from build123d import *

# Parameters (mm, degrees)
SKETCH2_W           = 102
SKETCH2_H           = 96.13
SKETCH2_W_2         = 92
SKETCH2_H_2         = 64.53
BOSS_EXTRUDE1_DEPTH = 85
SKETCH8_R           = 10.25
CUT_EXTRUDE7_DEPTH  = 20
SKETCH9_R           = 12.7
CUT_EXTRUDE8_DEPTH  = 20
SKETCH10_R          = 3.875
CUT_EXTRUDE9_DEPTH  = 142.206388754
SKETCH11_W          = 48.065
SKETCH11_H          = 85
CUT_EXTRUDE10_DEPTH = 142.206388754
SKETCH14_R          = 1.5
BOSS_EXTRUDE2_DEPTH = 10
SKETCH15_R          = 15.5
SKETCH15_R_2        = 12.7
BOSS_EXTRUDE3_DEPTH = 10
FILLET1_R           = 1.5
CUT_EXTRUDE11_DEPTH = 142.206388754


with BuildPart() as part:
    # Sketch2 → Boss-Extrude1 (new body)
    with BuildSketch(Plane(origin=(0, 0, 0), x_dir=(1, 0, 0), z_dir=(0, 1, 0))):
        Rectangle(SKETCH2_W, SKETCH2_H)
        Rectangle(SKETCH2_W_2, SKETCH2_H_2, mode=Mode.SUBTRACT)
    extrude(amount=BOSS_EXTRUDE1_DEPTH)

    # Sketch8 → Cut-Extrude7 (cut)
    with BuildSketch(Plane.XY.offset(48.065)):
        with Locations((-31, 31.7)):
            Circle(SKETCH8_R)
        with Locations((29, 31.7)):
            Circle(SKETCH8_R)
    extrude(amount=-CUT_EXTRUDE7_DEPTH, mode=Mode.SUBTRACT)

    # Sketch9 → Cut-Extrude8 (cut)
    with BuildSketch(Plane(origin=(0, 0, -48.065), x_dir=(-1, 0, 0), z_dir=(0, 0, -1))):
        with Locations((-12, 28.575)):
            Circle(SKETCH9_R)
        with Locations((29, 28.575)):
            Circle(SKETCH9_R)
    extrude(amount=-CUT_EXTRUDE8_DEPTH, mode=Mode.SUBTRACT)

    # Sketch10 → Cut-Extrude9 (cut, through all)
    with BuildSketch(Plane.ZY.offset(51)):
        with Locations((0, 28.575)):
            Circle(SKETCH10_R)
    extrude(amount=-CUT_EXTRUDE9_DEPTH, mode=Mode.SUBTRACT)

    # Sketch11 → Cut-Extrude10 (cut, through all)
    with BuildSketch(Plane.ZY.offset(51)):
        with Locations((24.0325, 42.5)):
            Rectangle(SKETCH11_W, SKETCH11_H)
    extrude(amount=-CUT_EXTRUDE10_DEPTH, mode=Mode.SUBTRACT)

    # Sketch14 → Boss-Extrude2 (add)
    with BuildSketch(Plane.XY):
        with Locations(Location((-48.5, 58.725, 0), (0, 0, 180))):
            Circle(SKETCH14_R)
        with Locations(Location((-48.5, 4.675, 0), (0, 0, 180))):
            Circle(SKETCH14_R)
        with Locations(Location((48.5, 4.675, 0), (0, 0, 180))):
            Circle(SKETCH14_R)
        with Locations(Location((48.5, 58.725, 0), (0, 0, 180))):
            Circle(SKETCH14_R)
    extrude(amount=BOSS_EXTRUDE2_DEPTH)

    # Sketch15 → Boss-Extrude3 (add)
    # profile 1 of 2: a face of its own
    with BuildSketch(Plane.XY.offset(-32.265)):
        with Locations((12, 28.575)):
            Circle(SKETCH15_R)
        with Locations(Location((12, 28.575, 0), (0, 0, 180))):
            Circle(SKETCH15_R_2, mode=Mode.SUBTRACT)
    # profile 2 of 2: a face of its own
    with BuildSketch(Plane.XY.offset(-32.265)):
        with Locations((-29, 28.575)):
            Circle(SKETCH15_R)
        with Locations(Location((-29, 28.575, 0), (0, 0, 180))):
            Circle(SKETCH15_R_2, mode=Mode.SUBTRACT)
    extrude(amount=BOSS_EXTRUDE3_DEPTH)

    # Fillet1
    fillet1_edges = [part.edges().sort_by_distance(p)[0] for p in [
        (24.7, 28.575, -22.265),
        (-16.3, 28.575, -22.265),
    ]]
    fillet(fillet1_edges, radius=FILLET1_R)

    # Sketch16 → Cut-Extrude11 (cut, through all)
    with BuildSketch(Plane.ZY.offset(51)):
        Polygon((-48.065, 6.5), (-45.236572875, 3.671572875), (-45.236572875, 9), (-48.065, 9), align=None)
    extrude(amount=-CUT_EXTRUDE11_DEPTH, mode=Mode.SUBTRACT)


solid = part.part
Work out the finished part from the listing and answer in its coordinate system (mm). A direction names the side the tool comes from. Round coordinates to 2 decimals unless told otherwise and drop trailing zeros. Loops run counter-clockwise (first coordinate to the right, second up) from the corner with the lowest first, then second, coordinate; pieces in that order, holes last. Notation, with made-up numbers: (-30, -40) - (18, -40) arc R23 ccw to (18, -5) - close; hole circle Ø10 at (17.5, 34). An arc over 180 degrees is marked (long way). Use one line per item in the form item = value. Start each with the question number.
(1) Find section B-B on x = 12. Determine the outline of the cut face in (y, z) (3 decimals), and give its area (3 significant figures).
(2) Consider line 1 (X direction, y = 6.5, z = -31); line 2 (Y direction, x = 12, z = -36.25) (3 decimals); line 3 (X direction, y = 21, z = -24.5). Determine where each line is inside the solid, lowest interval first.
(3) Which of the six approach directions +Z, -Z, +X, -X, +Y, -Y give full straight-line access (tool end or side, diameter ignored) to faces 1 (the face through (49.606, 57.711, 4.93)), 2 (the face through (-22, 16, -22.265)), 3 (the face through (-51, 42, -24))?
(4) Determine the mould class of faces 4 (the face through (-1, 9, -47)), 5 (the face through (-12, 0, -35)), 6 (the face through (-1, 3, -48.065)) for opening direction Y: +Y half, -Y half, draft (parallel to the pull), parting line (faces both ways), or undercut.
(5) Flat-ended cylindrical pins translate along their axes: P1, Ø1.5, axis at x = -49.5, y = 68.5, coming from the +Z side; P2, Ø5, axis at x = 6, y = 15, coming from the +Z side (3 decimals); P3, Ø3, axis at x = -32, y = 11.5, coming from the +Z side (3 decimals). Find the tip coordinate at first contact, or state that the pin passes through.
(6) Find section D-D on y = 74.5. Determine the outline of the cut face in (x, z) (3 decimals), and give its area (3 significant figures).
(7) Find section C-C on z = -20. Determine the outline of the cut face in (x, y), and give its area (3 significant figures).
(8) Find section A-A on z = -27. Determine the outline of the cut face in (x, y) (3 decimals).
Answer list:
q1.outline = (0, -48.065) - (6.5, -48.065) - (3.672, -45.237) - (9, -45.237) - (9, -48.065) - (15.875, -48.065) - (15.875, -23.765) arc R1.5 ccw to (14.375, -22.265) - (13.075, -22.265) - (13.075, -32.265) - (0, -32.265) - close; (41.275, -48.065) - (85, -48.065) - (85, -32.265) - (44.075, -32.265) - (44.075, -22.265) - (42.775, -22.265) arc R1.5 ccw to (41.275, -23.765) - close
q1.area = 986 mm^2
q2.line_1 = -51 to -46, 46 to 51
q2.line_2 = 0 to 15.875, 41.275 to 85
q2.line_3 = -51 to -46, -42.52 to -39.19, -18.81 to -15.48, -1.52 to 1.81, 22.19 to 25.52, 46 to 51
q3.face_1 = +Z
q3.face_2 = +Z, +Y, -Y
q3.face_3 = +Z, -Z, -X, +Y, -Y
q4.face_4 = undercut
q4.face_5 = -Y half
q4.face_6 = draft
q5.P1 = 0
q5.P2 = -22.265
q5.P3 = -32.265
q6.outline = (-51, -48.065) - (51, -48.065) - (51, 0) - (46, 0) - (46, -32.265) - (-46, -32.265) - (-46, 0) - (-51, 0) - close
q6.area = 1,930 mm^2
q7.outline = (-51, 0) - (-46, 0) - (-46, 85) - (-51, 85) - close; (46, 0) - (51, 0) - (51, 85) - (46, 85) - close
q7.area = 850 mm^2
q8.outline = (-51, 0) - (-46, 0) - (-46, 85) - (-51, 85) - close; circle Ø31 at (-29, 28.575); circle Ø31 at (12, 28.575); (46, 0) - (51, 0) - (51, 85) - (46, 85) - close; hole circle Ø25.4 at (-29, 28.575); hole circle Ø25.4 at (12, 28.575)
